Could you check a few things on this drawing? It's one solid part, dimensions in mm from its lowest x, y, z. A direction names the side the tool comes from. Round coordinates to 2 decimals unless told otherwise and drop trailing zeros. Write each loop counter-clockwise with the first axis right and the second up, starting at its lowest first coordinate (ties: lowest second). Pieces come first, ordered by that corner, then holes. Notation, with made-up numbers: (8.5, -21.75) -> (35.5, -21.75) arc R10 cw to (35.5, -9.75) -> close; hole circle Ø9 at (25, 72.25). An arc over 180 degrees is marked (long way). Put each result on its own line as item: value. Start each with the question number.
1) Will these pins go through, and if not, where does the flat tip stop? P1, Ø3, axis at x = 25.5, y = 3.5, coming from the +Z side; P2, Ø8, axis at x = 28.5, z = 32, coming from the -Y side; P3, Ø5.5, axis at x = 20, z = 23.85, coming from the -Y side; P4, Ø6, axis at x = 11, y = 9.5, coming from the +Z side.
2) I want a section at B-B, the plane y = 18. List the corners of the cut face in (x, z) for me, then the cut area to 3 significant figures.
3) We'd pull the mould along X, two halves only. Please class the marked faces 3, 4, 5 and 6: released by +X, released by -X, zero draft, split by the parting line, or undercut.
4) If I drill on line 1 along Y through (x, z) = (14.5, 22); line 2 along Z through (x, y) = (3, 10.5); line 3 along Z through (x, y) = (33, 17.5), over which ranges is the centre line in solid material (lowest first)? Write a range as [from, to].
5) Which directions (+Z, -Z, +X, -X, +Y, -Y) give clear straight access to the entire face, cutting with the end or side of a thin tool? Please do the marked faces 1 and 2.
6) I want a section at C-C, the plane z = 21.5. List the corners of the cut face in (x, y) for me, then the cut area to 3 significant figures.
7) I want a section at D-D, the plane x = 13. List the corners of the cut face in (y, z) for me.
8) I want a section at A-A, the plane x = 20. List the corners of the cut face in (y, z) for me.
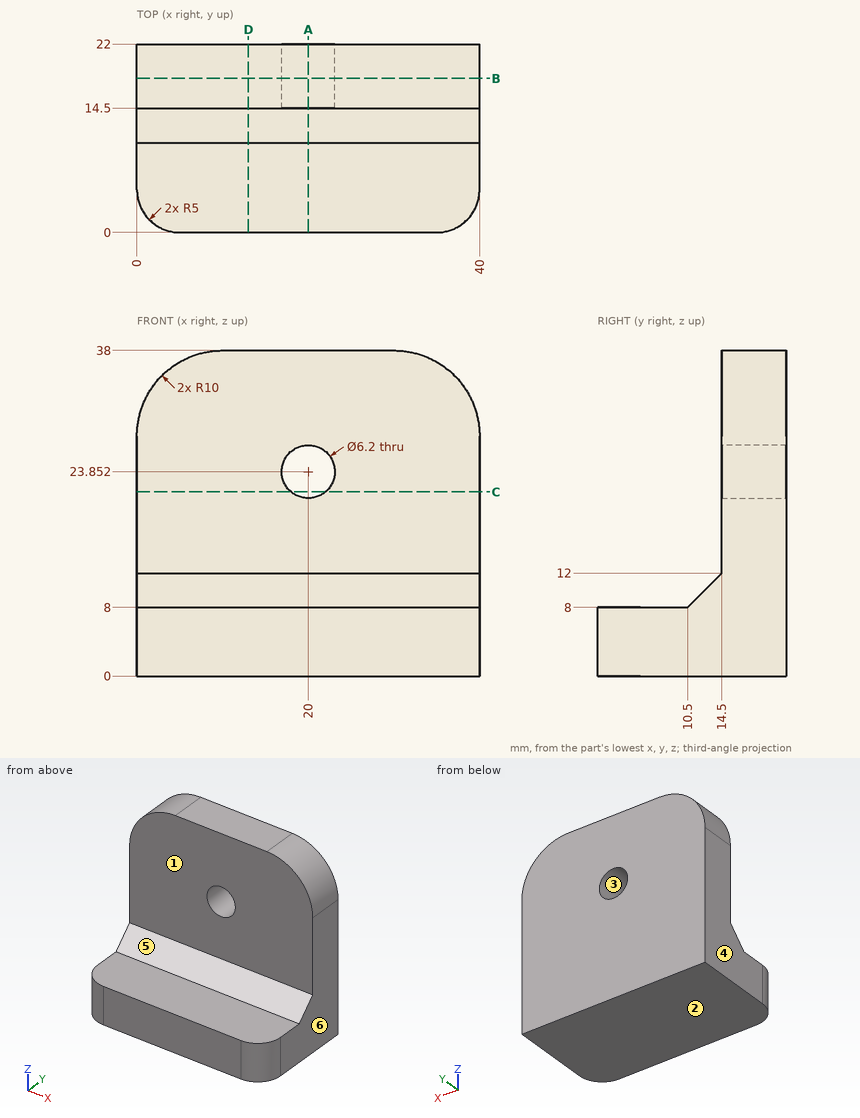
Findings:
1. P1: stops at z = 8
1. P2: stops at y = 14.5
1. P3: passes through
1. P4: stops at z = 10
2. outline: (0, 0) -> (40, 0) -> (40, 28) arc R10 ccw to (30, 38) -> (10, 38) arc R10 ccw to (0, 28) -> close; hole circle Ø6.2 at (20, 23.85)
2. area: 1,450 mm2
3. face 3: undercut
3. face 4: released by -X
3. face 5: zero draft
3. face 6: released by +X
4. line 1: y = [14.5, 22]
4. line 2: z = [0, 8]
4. line 3: z = [0, 37.54]
5. face 1: +Z, +X, -X, -Y
5. face 2: -Z, +X, -X, +Y, -Y
6. outline: (0, 14.5) -> (17.98, 14.5) -> (17.98, 22) -> (0, 22) -> close; (22.02, 14.5) -> (40, 14.5) -> (40, 22) -> (22.02, 22) -> close
6. area: 270 mm2
7. outline: (0, 0) -> (22, 0) -> (22, 38) -> (14.5, 38) -> (14.5, 12) -> (10.5, 8) -> (0, 8) -> close
8. outline: (0, 0) -> (22, 0) -> (22, 20.75) -> (14.5, 20.75) -> (14.5, 12) -> (10.5, 8) -> (0, 8) -> close; (14.5, 26.95) -> (22, 26.95) -> (22, 38) -> (14.5, 38) -> close
